Could you check a few things on this model? Use its own coordinates, in mm. Coordinates: 2 decimals unless noted, no trailing zeros. Put each result on its own line as item: value. Start each with the question number.
Q1. Please list where these lines run through material, in increasing order: line 1 along Z through (x, y) = (-30, -0.35); line 2 along Z through (x, y) = (-79.5, -0.1); line 3 along Z through (x, y) = (21.5, -0.1).
Q2. If we section it at A-A (z = -49.5): Count the separate pieces of the cut face and the enclosed holes in it, and give its area (3 significant figures).
Q3. Will this pin go through, and if not, where does the flat tip stop? pin 1 (9 mm diameter, centred on x = 30.18, z = -6.34, fed in from -Y).
from build123d import *

# Parameters (mm, degrees)
SKETCH1_W               = 203.2
SKETCH1_H               = 101.6
BOSS_EXTRUDE2_DEPTH     = 0.762
CUT_EXTRUDE1_DEPTH      = 118.861900687
CUT_EXTRUDE1_DEPTH_BACK = 118.861900687
SKETCH2_R               = 7.62


with BuildPart() as part:
    # Sketch1 → Boss-Extrude2 (new body)
    with BuildSketch(Plane(origin=(0, 0, 0), x_dir=(1, 0, 0), z_dir=(0, 1, 0))):
        with Locations((1.482009724, 6.339708266)):
            Rectangle(SKETCH1_W, SKETCH1_H)
    extrude(amount=-BOSS_EXTRUDE2_DEPTH)

    # Sketch2 → Cut-Extrude1 (cut, two sides: drawn at the far end of the back side and taken through both)
    with BuildSketch(Plane(origin=(0, 0, 0), x_dir=(1, 0, 0), z_dir=(0, 1, 0)).offset(-CUT_EXTRUDE1_DEPTH_BACK)):
        with Locations(Location((90.382009724, -31.760291734, 0), (0, 0, 270))):
            Circle(SKETCH2_R)
        with Locations(Location((90.382009724, 6.339708266, 0), (0, 0, 270))):
            Circle(SKETCH2_R)
        with Locations(Location((90.382009724, 44.439708266, 0), (0, 0, 270))):
            Circle(SKETCH2_R)
        with Locations(Location((70.316009724, -31.760291734, 0), (0, 0, 270))):
            Circle(SKETCH2_R)
        with Locations(Location((50.250009724, -31.760291734, 0), (0, 0, 270))):
            Circle(SKETCH2_R)
        with Locations(Location((30.184009724, -31.760291734, 0), (0, 0, 270))):
            Circle(SKETCH2_R)
        with Locations(Location((10.118009724, -31.760291734, 0), (0, 0, 270))):
            Circle(SKETCH2_R)
        with Locations(Location((-9.947990276, -31.760291734, 0), (0, 0, 270))):
            Circle(SKETCH2_R)
        with Locations(Location((-30.013990276, -31.760291734, 0), (0, 0, 270))):
            Circle(SKETCH2_R)
        with Locations(Location((-50.079990276, -31.760291734, 0), (0, 0, 270))):
            Circle(SKETCH2_R)
        with Locations(Location((-70.145990276, -31.760291734, 0), (0, 0, 270))):
            Circle(SKETCH2_R)
        with Locations(Location((-90.211990276, -31.760291734, 0), (0, 0, 270))):
            Circle(SKETCH2_R)
        with Locations(Location((70.316009724, 6.339708266, 0), (0, 0, 270))):
            Circle(SKETCH2_R)
        with Locations(Location((50.250009724, 6.339708266, 0), (0, 0, 270))):
            Circle(SKETCH2_R)
        with Locations(Location((30.184009724, 6.339708266, 0), (0, 0, 270))):
            Circle(SKETCH2_R)
        with Locations(Location((10.118009724, 6.339708266, 0), (0, 0, 270))):
            Circle(SKETCH2_R)
        with Locations(Location((-9.947990276, 6.339708266, 0), (0, 0, 270))):
            Circle(SKETCH2_R)
        with Locations(Location((-30.013990276, 6.339708266, 0), (0, 0, 270))):
            Circle(SKETCH2_R)
        with Locations(Location((-50.079990276, 6.339708266, 0), (0, 0, 270))):
            Circle(SKETCH2_R)
        with Locations(Location((-70.145990276, 6.339708266, 0), (0, 0, 270))):
            Circle(SKETCH2_R)
        with Locations(Location((-90.211990276, 6.339708266, 0), (0, 0, 270))):
            Circle(SKETCH2_R)
        with Locations(Location((70.316009724, 44.439708266, 0), (0, 0, 270))):
            Circle(SKETCH2_R)
        with Locations(Location((50.250009724, 44.439708266, 0), (0, 0, 270))):
            Circle(SKETCH2_R)
        with Locations(Location((30.184009724, 44.439708266, 0), (0, 0, 270))):
            Circle(SKETCH2_R)
        with Locations(Location((10.118009724, 44.439708266, 0), (0, 0, 270))):
            Circle(SKETCH2_R)
        with Locations(Location((-9.947990276, 44.439708266, 0), (0, 0, 270))):
            Circle(SKETCH2_R)
        with Locations(Location((-30.013990276, 44.439708266, 0), (0, 0, 270))):
            Circle(SKETCH2_R)
        with Locations(Location((-50.079990276, 44.439708266, 0), (0, 0, 270))):
            Circle(SKETCH2_R)
        with Locations(Location((-70.145990276, 44.439708266, 0), (0, 0, 270))):
            Circle(SKETCH2_R)
        with Locations(Location((-90.211990276, 44.439708266, 0), (0, 0, 270))):
            Circle(SKETCH2_R)
        with Locations(Location((80.349009724, -12.710291734, 0), (0, 0, 270))):
            Circle(SKETCH2_R)
        with Locations(Location((80.349009724, 25.389708266, 0), (0, 0, 270))):
            Circle(SKETCH2_R)
        with Locations(Location((60.283009724, -12.710291734, 0), (0, 0, 270))):
            Circle(SKETCH2_R)
        with Locations(Location((60.283009724, 25.389708266, 0), (0, 0, 270))):
            Circle(SKETCH2_R)
        with Locations(Location((40.217009724, -12.710291734, 0), (0, 0, 270))):
            Circle(SKETCH2_R)
        with Locations(Location((40.217009724, 25.389708266, 0), (0, 0, 270))):
            Circle(SKETCH2_R)
        with Locations(Location((20.151009724, -12.710291734, 0), (0, 0, 270))):
            Circle(SKETCH2_R)
        with Locations(Location((20.151009724, 25.389708266, 0), (0, 0, 270))):
            Circle(SKETCH2_R)
        with Locations(Location((0.085009724, -12.710291734, 0), (0, 0, 270))):
            Circle(SKETCH2_R)
        with Locations(Location((0.085009724, 25.389708266, 0), (0, 0, 270))):
            Circle(SKETCH2_R)
        with Locations(Location((-19.980990276, -12.710291734, 0), (0, 0, 270))):
            Circle(SKETCH2_R)
        with Locations(Location((-19.980990276, 25.389708266, 0), (0, 0, 270))):
            Circle(SKETCH2_R)
        with Locations(Location((-40.046990276, -12.710291734, 0), (0, 0, 270))):
            Circle(SKETCH2_R)
        with Locations(Location((-40.046990276, 25.389708266, 0), (0, 0, 270))):
            Circle(SKETCH2_R)
        with Locations(Location((-60.112990276, -12.710291734, 0), (0, 0, 270))):
            Circle(SKETCH2_R)
        with Locations(Location((-60.112990276, 25.389708266, 0), (0, 0, 270))):
            Circle(SKETCH2_R)
        with Locations(Location((-80.178990276, -12.710291734, 0), (0, 0, 270))):
            Circle(SKETCH2_R)
        with Locations(Location((-80.178990276, 25.389708266, 0), (0, 0, 270))):
            Circle(SKETCH2_R)
    extrude(amount=CUT_EXTRUDE1_DEPTH + CUT_EXTRUDE1_DEPTH_BACK, mode=Mode.SUBTRACT)


solid = part.part
The answers:
1. line 1: -57.14 to -52.06, -36.82 to -13.96, 1.28 to 24.14, 39.38 to 44.46
1. line 2: -57.14 to -32.98, -17.8 to 5.12, 20.3 to 44.46
1. line 3: -57.14 to -32.89, -17.89 to 5.21, 20.21 to 44.46
2. separate pieces: 11
2. enclosed holes: 0
2. area: 68.0 mm^2
3. pin 1: through
